Could you check a few things on this drawing? It's one solid part, dimensions in mm from its lowest x, y, z. A direction names the side the tool comes from. Round coordinates to 2 decimals unless told otherwise and drop trailing zeros. Loops run counter-clockwise (first coordinate to the right, second up) from the corner with the lowest first, then second, coordinate; pieces in that order, holes last. Notation, with made-up numbers: M -8,65 L 13,65 A21 ccw 13,72 Z; hole C 68.25,-26 d10. An arc over 180 degrees is marked long. Return JSON: item names as keys, results as strings.
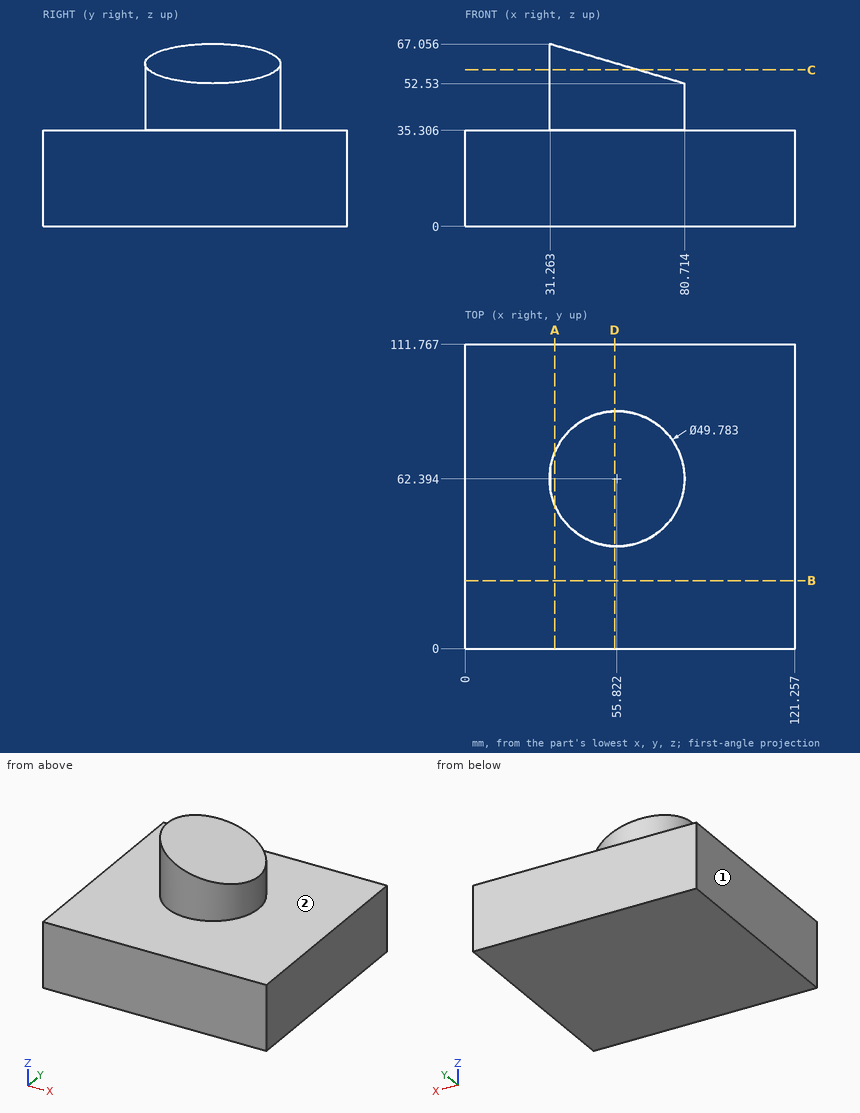
Q1. If I drill on line 1 along Z through (x, y) = (51.5, 18); line 2 along Y through (x, z) = (65.5, 42); line 3 along Z through (x, y) = (66, 40), over which ranges is the centre line in solid material (lowest first)?
Results:
{"line 1": "z = 0 to 35.31", "line 2": "y = 39.46 to 85.33", "line 3": "z = 0 to 56.85"}
Q2. I'm going to push flat-ended pins straight in: pin 1 Ø12 at (x, z) = (43, 59.5) entering from -Y (1 decimal); pin 2 Ø12 at (x, y) = (23, 32) entering from +Z; pin 3 Ø5 at (x, y) = (68, 71) entering from +Z. Where does each tip first touch, or does it pass through?
Results:
{"pin 1": "stops at y = 38.5", "pin 2": "stops at z = 35.31", "pin 3": "stops at z = 57"}
Q3. Suppose I cut it at A-A, the plane x = 33. Please give me the cut outline in (y, z) (1 decimal).
Results:
{"outline": "M 0,0 L 111.8,0 L 111.8,35.3 L 72.3,35.3 L 72.3,66.5 L 52.5,66.5 L 52.5,35.3 L 0,35.3 Z"}
Q4. Suppose I cut it at C-C, the plane z = 57.5. Please give me the cut outline in (x, y) (1 decimal).
Results:
{"outline": "M 63.8,38.8 L 63.8,86 A24.9 ccw long Z"}
Q5. Suppose I cut it at B-B, the plane y = 25. Please give me the cut outline in (x, z).
Results:
{"outline": "M 0,0 L 121.26,0 L 121.26,35.31 L 0,35.31 Z"}
Q6. On a 3-axis mill with a long thin cutter (end or side, diameter ignored), from which of +Z, -Z, +X, -X, +Y, -Y can I reach the whole of each face in a straight line? I mean the marked faces 1 and 2. Say none if no direction works.
Results:
{"face 1": "+Z, -Z, -X, +Y, -Y", "face 2": "+Z"}
Q7. Suppose I cut it at D-D, the plane x = 55. Please give me the cut outline in (y, z), plus the area to 3 significant figures.
Results:
{"outline": "M 0,0 L 111.77,0 L 111.77,35.31 L 87.27,35.31 L 87.27,60.08 L 37.52,60.08 L 37.52,35.31 L 0,35.31 Z", "area": "5,180 mm2"}
